CAD build for the part. Positions are in the model's coordinates, mm. A direction names the side the tool comes from. Coordinates: 2 decimals unless noted, no trailing zeros. Write each loop counter-clockwise with the first axis right and the second up, starting at its lowest first coordinate (ties: lowest second). Pieces come first, ordered by that corner, then holes. Notation, with made-up numbers: (77, 5.25) - (114, 5.25) arc R23 ccw to (114, 22.25) - close; hole circle Ø8 at (-8.75, 32). An arc over 180 degrees is marked (long way). Answer in a Markdown table with one row per item. Add a question column.
Q1. Drill centre lines: line 1 along X through (y, z) = (13.45, -3.81) (3 decimals); line 2 along Z through (x, y) = (14.25, 14.5) (3 decimals); line 3 along Y through (x, z) = (10.75, -7). Where is each one in solid material? Low to high. Write a range as from..to.
Q2. 3-axis set-ups, long thin cutter, end or side, ignore diameter. For faces 1 (the flat face through (11, 13, 1.905)), 2 (the cylindrical face through (12.4, 13.1, -5)), 3 (the cylindrical face through (-6.59, 9.69, -8.55)), 4 (the flat face through (-7.4, 10.478, 0.2)): which of +Z, -Z, +X, -X, +Y, -Y reach the whole face in a straight line?
Q3. Two-plate mould, pull along X, no slides. Class faces 5 (the flat face through (10, 10.478, -3)), 6 (the flat face through (0, 10, 9)), 7 (the flat face through (0, 13, -9)): +X half, -X half, draft (parallel to the pull), parting line (faces both ways), or undercut.
Q4. Band-saw the part on B-B (y = 4.25). List the corners of the cut face in (x, z) (3 decimals), and give its area (3 significant figures).
Q5. Band-saw the part on D-D (z = -3). List the corners of the cut face in (x, y) (1 decimal), and give its area (3 significant figures).
Q6. Band-saw the part on C-C (x = 3.5). List the corners of the cut face in (y, z) (1 decimal).
Q7. Pin check, flat tips, straight feed: pin 1 (2 mm diameter, centred on x = 11, y = 13, fed in from +Z) (3 decimals); pin 2 (6.5 mm diameter, centred on x = 10.795, z = -3.81, fed in from -Y); pin 3 (2.5 mm diameter, centred on y = 13.5, z = -9, fed in from -X). Stop position of each tip, or through.
```python
from build123d import *

# Parameters (mm, degrees)
SKETCH2_W           = 5.23875
SKETCH2_H           = 6.95
SKETCH2_W_2         = 1.5875
SKETCH2_H_2         = 3.845
SKETCH2_W_3         = 17.78
SKETCH3_R           = 11.338051479
CUT_EXTRUDE1_DEPTH  = 21.336
SKETCH5_R           = 1.75
CUT_EXTRUDE3_DEPTH  = 27.432
BOSS_EXTRUDE2_START = -5.23875
SKETCH5_3_R         = 2
BOSS_EXTRUDE2_DEPTH = 5.23875
FILLET1_R           = 0.79375
CUT_EXTRUDE4_START  = -14.224
CUT_EXTRUDE4_DEPTH  = 14.224
FILLET2_R           = 0.79375


with BuildPart() as part:
    # Sketch2 → Revolve2 (revolve)
    with BuildSketch(Plane(origin=(0, 0, 0), x_dir=(0, 1, 0), z_dir=(0, 0, 1)), mode=Mode.PRIVATE) as revolve2_sk:
        with Locations((-13.096875, 3.475)):
            Rectangle(SKETCH2_W, SKETCH2_H)
        with Locations((-9.68375, 3.475)):
            Rectangle(SKETCH2_W_2, SKETCH2_H)
        with Locations((-9.68375, 8.8725)):
            Rectangle(SKETCH2_W_2, SKETCH2_H_2)
        with Locations((0, 3.475)):
            Rectangle(SKETCH2_W_3, SKETCH2_H)
        with Locations((9.68375, 3.475)):
            Rectangle(SKETCH2_W_2, SKETCH2_H)
        with Locations((9.68375, 8.8725)):
            Rectangle(SKETCH2_W_2, SKETCH2_H_2)
        with Locations((13.096875, 3.475)):
            Rectangle(SKETCH2_W, SKETCH2_H)
    revolve(revolve2_sk.sketch.rotate(Axis((0, -15.71625, 0), (0, 1, 0)), 180), axis=Axis((0, -15.71625, 0), (0, 1, 0)))

    # Sketch3 → Cut-Extrude1 (cut)
    with BuildSketch(Plane(origin=(0, 0, 0), x_dir=(-1, 0, 0), z_dir=(0, 1, 0))):
        Circle(SKETCH3_R)
    extrude(amount=-CUT_EXTRUDE1_DEPTH, mode=Mode.SUBTRACT)

    # Sketch5 → Cut-Extrude3 (cut)
    with BuildSketch(Plane(origin=(0, 15.71625, 0), x_dir=(-1, 0, 0), z_dir=(0, 1, 0))):
        with Locations((-3.175, 0)):
            Circle(SKETCH5_R)
    extrude(amount=-CUT_EXTRUDE3_DEPTH, mode=Mode.SUBTRACT)

    # Sketch5<3> → Boss-Extrude2 (add)
    with BuildSketch(Plane(origin=(0, 15.71625, 0), x_dir=(-1, 0, 0), z_dir=(0, 1, 0)).offset(BOSS_EXTRUDE2_START)):
        with BuildLine():
            Line((-15.875, -10.795), (0, -10.795))
            Line((0, -10.795), (0, -6.95))
            ThreePointArc((0, -6.95), (-5.547172703, -4.187048483), (-6.683821886, 1.905))
            Line((-6.683821886, 1.905), (-15.875, 1.905))
            Line((-15.875, 1.905), (-15.875, -10.795))
        make_face()
        with Locations((-10.795, -3.81)):
            Circle(SKETCH5_3_R, mode=Mode.SUBTRACT)
    extrude(amount=BOSS_EXTRUDE2_DEPTH)

    # Fillet1
    # the kernel refuses this fillet: 0.79375 mm, written as the material it adds along each edge
    with BuildSketch(Plane(origin=(0, 10.4775, -6.95), x_dir=(-0.9986823309895368, 0, 0.051318629846335534), z_dir=(0, 1, 0))) as fillet1_piece_1:
        with BuildLine():
            CenterArc((0.754063117, -0.7927041), FILLET1_R, 92.941633047, 84.116733906)
            Line((-0.038640983, -0.751969938), (0, 0))
            ThreePointArc((0, 0), (0.356664477, -0.0091578), (0.713328955, 0))
        make_face()
    extrude(amount=5.23875)
    with BuildSketch(Plane(origin=(6.683821886, 9.041391923, 1.905), x_dir=(1, 0, 0), z_dir=(0, 1, 0))) as fillet1_piece_2:
        with BuildLine():
            CenterArc((0.574443231, -0.79375), FILLET1_R, 90, 69.603984808)
            ThreePointArc((-0.169543589, -0.51712268), (-0.079708314, -0.26022145), (0, 0))
            Line((0, 0), (0.574443231, 0))
        make_face()
    extrude(amount=6.674858077)
    # the kernel refuses this fillet: 0.79375 mm, written as the material it takes off along each edge
    with BuildSketch(Plane(origin=(0, 10.4775, -10.795), x_dir=(1, 0, 0), z_dir=(0, 1, 0))) as fillet1_2_piece_1:
        with BuildLine():
            CenterArc((FILLET1_R, -FILLET1_R), FILLET1_R, 90, 90)
            Line((0, -FILLET1_R), (0, 0))
            Line((0, 0), (FILLET1_R, 0))
        make_face()
    extrude(amount=7.223125, mode=Mode.SUBTRACT)
    with BuildSketch(Plane(origin=(15.875, 8.493125, 1.905), x_dir=(0, 0, -1), z_dir=(0, 1, 0)), Plane(origin=(15.875, 8.493125, -10.795), x_dir=(-1, 0, 0), z_dir=(0, 1, 0))) as fillet1_2_piece_2:
        with BuildLine():
            CenterArc((FILLET1_R, FILLET1_R), FILLET1_R, 180, 90)
            Line((0, FILLET1_R), (0, 0))
            Line((0, 0), (FILLET1_R, 0))
        make_face()
    extrude(amount=9.2075, mode=Mode.SUBTRACT)

    # Sketch6 → Cut-Extrude4 (cut)
    with BuildSketch(Plane(origin=(0, 10.4775, 0), x_dir=(-1, 0, 0), z_dir=(0, 1, 0)).offset(CUT_EXTRUDE4_START)):
        with BuildLine():
            ThreePointArc((-6.514278297, 2.42212268), (-3.966657748, 5.70684907), (0, 6.95))
            Line((0, 6.95), (0, 10.795))
            ThreePointArc((0, 10.795), (-6.927032193, 8.279387055), (-10.625582337, 1.905))
            Line((-10.625582337, 1.905), (-7.258265116, 1.905))
            ThreePointArc((-7.258265116, 1.905), (-6.805238557, 2.046978568), (-6.514278297, 2.42212268))
        make_face()
    extrude(amount=CUT_EXTRUDE4_DEPTH, mode=Mode.SUBTRACT)

    # Fillet2
    # the kernel refuses this fillet: 0.79375 mm, written as the material it adds along each edge
    with BuildSketch(Plane(origin=(0, 8.89, 6.95), x_dir=(0.9986823309895368, 0, -0.05131862984633391), z_dir=(0, 1, 0))) as fillet2_piece_1:
        with BuildLine():
            CenterArc((0.754063117, -0.7927041), FILLET2_R, 92.941633047, 84.116733906)
            Line((-0.038640983, -0.751969938), (0, 0))
            ThreePointArc((0, 0), (0.356664477, -0.0091578), (0.713328955, 0))
        make_face()
    extrude(amount=1.5875)
    # the kernel refuses this fillet: 0.79375 mm, written as the material it takes off along each edge
    with BuildSketch(Plane(origin=(0, 6.746443854, 10.795), x_dir=(0, 0, -1), z_dir=(0, 1, 0))) as fillet2_2_piece_1:
        with BuildLine():
            CenterArc((0.825297773, 0.79375), FILLET2_R, 175.447928579, 94.552071421)
            ThreePointArc((0.034051564, 0.856746032), (0.00851625, 0.428711229), (0, 0))
            Line((0, 0), (0.825297773, 0))
        make_face()
    extrude(amount=5.874612291, mode=Mode.SUBTRACT)
    with BuildSketch(Plane(origin=(10.625582337, 7.107567927, 1.905), x_dir=(-1, 0, 0), z_dir=(0, 1, 0))) as fillet2_2_piece_2:
        with BuildLine():
            CenterArc((0.686260177, -0.79375), FILLET2_R, 90, 83.620629792)
            ThreePointArc((-0.102574915, -0.705555556), (-0.057113988, -0.351930706), (0, 0))
            Line((0, 0), (0.686260177, 0))
        make_face()
    extrude(amount=3.369932073, mode=Mode.SUBTRACT)


solid = part.part
```
Checked values:
| question | item | result |
|---|---|---|
| 1 | line 1 | x = -5.813..8.795, 12.795..15.875 |
| 1 | line 2 | z = -10.795..1.905 |
| 1 | line 3 | y = 10.48..15.72 |
| 2 | face 1 | +Z, +X, +Y, -Y |
| 2 | face 2 | +Y |
| 2 | face 3 | -Y |
| 2 | face 4 | -X, +Y |
| 3 | face 5 | undercut |
| 3 | face 6 | +X half |
| 3 | face 7 | -X half |
| 4 | outline | circle Ø13.9 at (0, 0); hole circle Ø3.5 at (3.175, 0) |
| 4 | area | 142 mm² |
| 5 | outline | (-10.4, 8.9) - (-6.3, 8.9) - (-6.3, 0) - (6.3, 0) - (6.3, 8.9) - (10.4, 8.9) - (10.4, 10.5) - (9, 10.5) - (9, 15.7) - (-6.3, 15.7) - (-6.3, 10.5) - (-10.4, 10.5) - close; (12.6, 10.5) - (15.9, 10.5) - (15.9, 15.7) - (12.6, 15.7) - close |
| 5 | area | 241 mm² |
| 6 | outline | (0, -6) - (8.9, -6) - (8.9, -10.2) - (10.5, -10.2) - (10.5, -10.8) - (15.7, -10.8) - (15.7, -1.7) - (0, -1.7) - close; (0, 1.7) - (15.7, 1.7) - (15.7, 6) - (0, 6) - close |
| 7 | pin 1 | stops at z = 1.905 |
| 7 | pin 2 | stops at y = 8.89 |
| 7 | pin 3 | stops at x = 0 |
